```python
from build123d import *

# Parameters (mm, degrees)
EXTRUDE_1_DEPTH     = 6
CUT_EXTRUDE_1_DEPTH = 79.531840676
CUT_EXTRUDE_2_DEPTH = 79.531840676
FILLET_1_R          = 2
M3X0_51_D           = 2.5
M3X0_51_DEPTH       = 8.5
M3X0_51_TIP         = 0.751075774


with BuildPart() as part:
    # Эскиз1 → Бобышка-Вытянуть1 (new body)
    with BuildSketch(Plane(origin=(0, 0, 0), x_dir=(1, 0, 0), z_dir=(0, 1, 0))):
        with BuildLine():
            Line((-22.5, 0), (-22.5, -75))
            Line((-22.5, -75), (22.5, -75))
            Line((22.5, -75), (22.5, 0))
            ThreePointArc((22.5, 0), (0, 22.5), (-22.5, 0))
        make_face()
    extrude(amount=EXTRUDE_1_DEPTH)

    # Эскиз2 → Вырез-Вытянуть1 (cut, through all)
    with BuildSketch(Plane(origin=(0, 6, 0), x_dir=(1, 0, 0), z_dir=(0, 1, 0))):
        with BuildLine():
            Line((-10.274368671, 12.374368671), (-10.274368671, -65))
            ThreePointArc((-10.274368671, -65), (-12.374368671, -67.1), (-14.474368671, -65))
            Line((-14.474368671, -65), (-14.474368671, 12.374368671))
            ThreePointArc((-14.474368671, 12.374368671), (-12.374368671, 14.474368671), (-10.274368671, 12.374368671))
        make_face()
        with BuildLine():
            Line((10.274368671, 12.374368671), (10.274368671, -65))
            ThreePointArc((10.274368671, -65), (12.374368671, -67.1), (14.474368671, -65))
            Line((14.474368671, -65), (14.474368671, 12.374368671))
            ThreePointArc((14.474368671, 12.374368671), (12.374368671, 14.474368671), (10.274368671, 12.374368671))
        make_face()
    extrude(amount=-CUT_EXTRUDE_1_DEPTH, mode=Mode.SUBTRACT)

    # Эскиз11 → Вырез-Вытянуть2 (cut, through all)
    with BuildSketch(Plane(origin=(0, 6, 0), x_dir=(1, 0, 0), z_dir=(0, 1, 0))):
        with BuildLine():
            Line((6.274368671, 18.5), (-6.274368671, 11.254983118))
            Line((-6.274368671, 11.254983118), (-6.274368671, 18.5))
            ThreePointArc((-6.274368671, 18.5), (0, 19.535037809), (6.274368671, 18.5))
        make_face()
        Polygon((-6.274368671, 6.266676792), (6.274368671, 13.511693674), (6.274368671, -0.97834009), align=None)
        Polygon((-6.274368671, 1.278370466), (6.274368671, -5.966646416), (-6.274368671, -13.211663298), align=None)
        Polygon((-6.274368671, -18.199969624), (6.274368671, -10.954952742), (6.274368671, -25.444986506), align=None)
        Polygon((-6.274368671, -23.18827595), (6.274368671, -30.433292832), (-6.274368671, -37.678309714), align=None)
        Polygon((-6.274368671, -42.66661604), (6.274368671, -35.421599157), (6.274368671, -49.911632922), align=None)
        Polygon((-6.274368671, -47.654922365), (6.274368671, -54.899939248), (-6.274368671, -62.14495613), align=None)
        Polygon((-6.274368671, -67.133262455), (6.274368671, -67.133262455), (6.274368671, -59.888245573), align=None)
    extrude(amount=-CUT_EXTRUDE_2_DEPTH, mode=Mode.SUBTRACT)

    # Скругление1
    fillet_1_edges = [part.edges().sort_by_distance(p)[0] for p in [
        (-6.274368671, 3, 62.14495613),
        (-6.274368671, 3, 47.654922365),
        (6.274368671, 3, 54.899939248),
        (-6.274368671, 3, 67.133262455),
        (6.274368671, 3, 59.888245573),
        (6.274368671, 3, 67.133262455),
        (-6.274368671, 3, -18.5),
        (6.274368671, 3, -18.5),
        (-6.274368671, 3, -11.254983118),
        (6.274368671, 3, 0.97834009),
        (-6.274368671, 3, -6.266676792),
        (6.274368671, 3, -13.511693674),
        (-6.274368671, 3, 13.211663298),
        (-6.274368671, 3, -1.278370466),
        (6.274368671, 3, 5.966646416),
        (6.274368671, 3, 25.444986506),
        (-6.274368671, 3, 18.199969624),
        (6.274368671, 3, 10.954952742),
        (-6.274368671, 3, 37.678309714),
        (-6.274368671, 3, 23.18827595),
        (6.274368671, 3, 30.433292832),
        (6.274368671, 3, 49.911632922),
        (-6.274368671, 3, 42.66661604),
        (6.274368671, 3, 35.421599157),
    ]]
    fillet(fillet_1_edges, radius=FILLET_1_R)

    # Отверстие обработанное метчиком M3x0.51
    with Locations(Plane.XY.offset(75)):
        with Locations((-13.5, 3), (-4.5, 3), (4.5, 3), (13.5, 3)):
            Hole(M3X0_51_D / 2, depth=M3X0_51_DEPTH)
            with Locations((0, 0, -(M3X0_51_DEPTH + M3X0_51_TIP / 2))):  # 118° drill point
                Cone(0, M3X0_51_D / 2, M3X0_51_TIP, mode=Mode.SUBTRACT)


solid = part.part
```
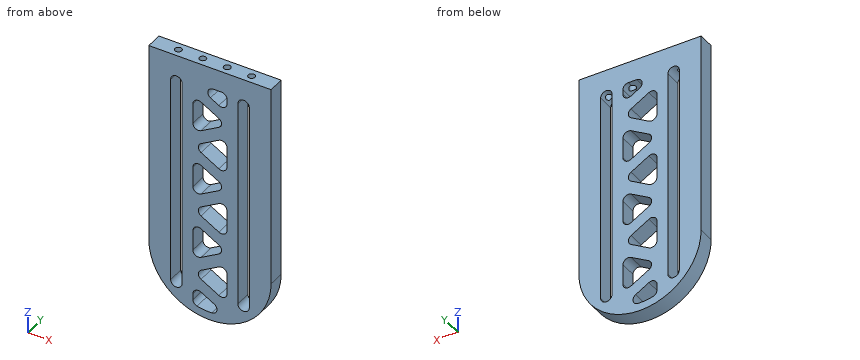
For this review, take the finished solid that the model builds, in its own axes (mm). Round coordinates to 2 decimals unless told otherwise and drop trailing zeros. Write each loop counter-clockwise with the first axis right and the second up, starting at its lowest first coordinate (ties: lowest second). Pieces come first, ordered by that corner, then holes. Notation, with made-up numbers: (-23, 27) - (-19, 27) arc R19 ccw to (-19, 36) - close; hole circle Ø8 at (44.5, -28). An arc over 180 degrees is marked (long way). Answer as a JSON object with one key per item and string values.
1. For pin 1 Ø2 at (x, y) = (11, 2.5) entering from -Z; pin 2 Ø3 at (x, y) = (-4.5, 3) entering from -Z; pin 3 Ø0.9 at (x, y) = (3, 2.5) entering from -Z, all flat-tipped, find the tip position at first contact; note any pin that passes through.
Response values:
{"pin 1": "stops at z = -20.16", "pin 2": "stops at z = -22.3", "pin 3": "stops at z = -22.36"}
2. We need section A-A on x = 18. Give the boundary of the cut face in (y, z).
Response values:
{"outline": "(0, -13.5) - (6, -13.5) - (6, 75) - (0, 75) - close"}
3. To check wall thickness, follow line 1 along X through (y, z) = (1.25, 17); line 2 along X through (y, z) = (3, 70.5); line 3 along X through (y, z) = (5.75, 30). State the ranges of each line that lie inside material, in increasing order.
Response values:
{"line 1": "x = -22.5 to -14.47, -10.27 to -3.87, 6.27 to 10.27, 14.47 to 22.5", "line 2": "x = -22.5 to -14.75, -12.25 to -5.75, -3.25 to 3.25, 5.75 to 12.25, 14.75 to 22.5", "line 3": "x = -22.5 to -14.47, -10.27 to -6.27, 4.23 to 10.27, 14.47 to 22.5"}
